Here's how the part is built. I have some questions about the finished solid (model axes, mm). Face numbers are marked on the shaded views. A direction names the side the tool comes from. Round coordinates to 2 decimals unless told otherwise and drop trailing zeros. Loops run counter-clockwise (first coordinate to the right, second up) from the corner with the lowest first, then second, coordinate; pieces in that order, holes last. Notation, with made-up numbers: M -36,28 L -15,28 A14 ccw -15,43 Z; hole C 75.25,-9.75 d4. An arc over 180 degrees is marked long. Answer as a JSON object with one key per item and string values.
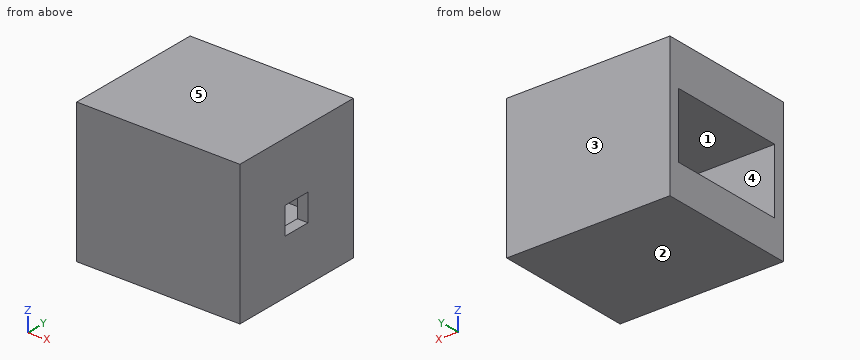
from build123d import *

# Parameters (mm, degrees)
F1_START      = 12.192
F1_DEPTH      = 7.808
F2_DEPTH      = 6.35
F3_DEPTH      = 20
F3_DEPTH_BACK = 6.35
F0_W          = 2
F0_H          = 5.2916666667
F4_DEPTH      = 6.35
F4_DEPTH_BACK = 3.81
F5_START      = 8.89
F5_DEPTH      = 11.11


with BuildPart() as f1:
    # F0 (on Top) → F1 (new body)
    with BuildSketch(Plane.XY.offset(F1_START)):
        Polygon((7.9375, 12.7), (-20.6375, 12.7), (-20.6375, -9.525), (7.9375, -9.525), (7.9375, -1.0583333333), (7.9375, 4.2333333333), align=None)
    extrude(amount=F1_DEPTH)



with BuildPart() as f2:
    # F0 (on Top) → F2 (new body)
    with BuildSketch(Plane.XY):
        Polygon((7.9375, 12.7), (-20.6375, 12.7), (-20.6375, -9.525), (7.9375, -9.525), (7.9375, -1.0583333333), (7.9375, 4.2333333333), align=None)
    extrude(amount=-F2_DEPTH)


with BuildPart() as f1_1:
    add(f1.part)

    add(f2.part)  # F3 merges F2
    # F0 (on Top) → F3 (join, two sides)
    with BuildSketch(Plane.XY) as f3_sk:
        Polygon((9.9375, 14.7), (-20.6375, 14.7), (-20.6375, 12.7), (7.9375, 12.7), (7.9375, 4.2333333333), (9.9375, 4.2333333333), align=None)
        Polygon((7.9375, -9.525), (-20.6375, -9.525), (-20.6375, -11.525), (9.9375, -11.525), (9.9375, -1.0583333333), (7.9375, -1.0583333333), align=None)
    extrude(amount=F3_DEPTH)
    extrude(f3_sk.sketch, amount=-F3_DEPTH_BACK)

    # F0 (on Top) → F4 (join, two sides)
    with BuildSketch(Plane.XY) as f4_sk:
        with Locations((8.9375, 1.5875)):
            Rectangle(F0_W, F0_H)
    extrude(amount=-F4_DEPTH)
    extrude(f4_sk.sketch, amount=F4_DEPTH_BACK)

    # F0 (on Top) → F5 (join)
    with BuildSketch(Plane.XY.offset(F5_START)):
        with Locations((8.9375, 1.5875)):
            Rectangle(F0_W, F0_H)
    extrude(amount=F5_DEPTH)


solid = f1_1.part
Item 1: I want a section at A-A on x = 0. List the corners of the cut face in (y, z) for me (3 decimals), plus the area to 3 significant figures.
Solution:
{"outline": "M -11.525,-6.35 L 14.7,-6.35 L 14.7,20 L -11.525,20 Z; hole M -9.525,0 L 12.7,0 L 12.7,12.192 L -9.525,12.192 Z", "area": "420 mm2"}
Item 2: I want a section at B-B on z = 3.25. List the corners of the cut face in (x, y) for me (1 decimal).
Solution:
{"outline": "M -20.6,-11.5 L 9.9,-11.5 L 9.9,14.7 L -20.6,14.7 L -20.6,12.7 L 7.9,12.7 L 7.9,-9.5 L -20.6,-9.5 Z"}
Item 3: If I drill on L1, parallel to Z at x = -8, y = -0.75; L2, parallel to Y at x = 2, z = 8.75 (3 decimals); L3, parallel to Y at x = 8.5, z = 5.5 (3 decimals), over which ranges is the centre line in solid material (lowest first)? Write a range as from..to.
Solution:
{"L1": "z = -6.35..0, 12.19..20", "L2": "y = -11.525..-9.525, 12.7..14.7", "L3": "y = -11.525..-1.058, 4.233..14.7"}
Item 4: We'd pull the mould along Z, two halves only. Please class the marked faces 1, 2 and 3: +Z half, -Z half, draft (parallel to the pull), parting line (faces both ways), or undercut.
Solution:
{"face 1": "undercut", "face 2": "-Z half", "face 3": "draft"}
Item 5: For the marked faces 4 and 5, which set-ups out of +Z, -Z, +X, -X, +Y, -Y let a thin tool reach every point of the face, with its end or its side?
Solution:
{"face 4": "-X", "face 5": "+Z, +X, -X, +Y, -Y"}
Item 6: I want a section at C-C on y = -6. List the corners of the cut face in (x, z) for me.
Solution:
{"outline": "M -20.64,-6.35 L 9.94,-6.35 L 9.94,20 L -20.64,20 L -20.64,12.19 L 7.94,12.19 L 7.94,0 L -20.64,0 Z"}
